CAD build for the part. Positions are in the model's coordinates, mm. A direction names the side the tool comes from. Round coordinates to 2 decimals unless told otherwise and drop trailing zeros. Loops run counter-clockwise (first coordinate to the right, second up) from the corner with the lowest first, then second, coordinate; pieces in that order, holes last. Notation, with made-up numbers: M 49,-23.5 L 96,-23.5 A31 ccw 96,15.5 Z; hole C -11,10.5 d7. An arc over 180 degrees is marked long. Use one line per item in the form item = value.
Autodesk Inventor part; units mm, degrees
ref_plane "YZ Plane" through (0, 0, 0) normal (1, 0, 0) x (0, 1, 0)
ref_plane "XZ Plane" through (0, 0, 0) normal (0, 1, 0) x (-1, 0, 0)
ref_plane "XY Plane" through (0, 0, 0) normal (0, 0, 1) x (1, 0, 0)
sketch "草圖1" plane through (0, 0, 0) normal (0, 0, 1) x (1, 0, 0)
  line L0 (-10, 120) -> (10, 120)
  line L1 (10, 120) -> (10, -20)
  line L2 (10, -20) -> (-10, -20)
  line L3 (-10, -20) -> (-10, 120)
  line L4 (10, 110) -> (-10, 110)
  line L5 (10, 120) -> (10, 110)
  line L6 (-10, 110) -> (-22, 110)
  line L7 (-22, 110) -> (-22, 120)
  line L8 (-22, 120) -> (-10, 120)
  line L9 (-10, 120) -> (-10, 110)
  line L10 (10, 110) -> (22, 110)
  line L11 (22, 110) -> (22, 120)
  line L12 (22, 120) -> (10, 120)
  line L13 (10, 120) -> (10, 110)
  point P0 (0, 0)
  point P1 (0, -20)
  dimension "d0" = 20
  dimension "d1" = 140
  dimension "d2" = 20
  dimension "d18" = 10
  dimension "d20" = 12
  dimension "d21" = 10
  dimension "d22" = 12
  dimension "d23" = 10
extrude "擠出1" add sketch "草圖1" along normal blind 10 contours L0 L1 L4 L3 | L3 L6 L7 L8 | L4 L1 L2 L3
sketch "草圖2" plane through (0, 0, 10) normal (0, 0, 1) x (1, 0, 0)
  circle A0 centre (0, 0) radius 10
  circle A1 centre (0, 0) radius 5
  dimension "d5" = 20
  dimension "d6" = 10
extrude "擠出2" add sketch "草圖2" along normal blind 10
sketch "草圖3" plane through (-10, 120, 0) normal (0, 1, 0) x (1, 0, 0)
  circle A0 centre (-2, -25) radius 10
  line L0 (20, -10) -> (-12, -10)
  line L1 (-12, 0) -> (20, 0)
  line L2 (-12, 0) -> (8, 0)
  line L3 (8, 0) -> (8, -25)
  line L4 (8, -25) -> (-12, -25)
  line L5 (-12, -25) -> (-12, 0)
  line L6 (-12, 0) -> (-12, -10)
  point P0 (10, 0)
  point P1 (0, -10)
  point P2 (0, 0)
  point P3 (32, -10)
  point P4 (32, 0)
  point P5 (8, -10)
  dimension "d9" = 20
  dimension "d10" = 25
extrude "擠出3" add sketch "草圖3" against normal blind 10 contours L4 A0 | A0 L5 L0 L3 | A0 L4
sketch "草圖4" plane through (-10, 120, 0) normal (0, 1, 0) x (1, 0, 0)
  circle A0 centre (-2, -25) radius 10
  circle A1 centre (-2, -25) radius 5
  point P0 (10, 0)
  point P1 (8, -25)
  point P2 (-12, -25)
  point P3 (0, 25)
  dimension "d13" = 10
extrude "擠出4" cut sketch "草圖4" against normal blind 10 contours A1
sketch "草圖5" plane through (0, 0, 10) normal (0, 0, 1) x (1, 0, 0)
  arc A0 (-10, 0) -> (10, 0) centre (0, 0) ccw
  line L0 (-10, 0) -> (-10, -20)
  line L1 (-10, -20) -> (10, -20)
  line L2 (10, -20) -> (10, 0)
extrude "擠出5" cut sketch "草圖5" against normal through all
equation "\"d21\" = d18"
equation "\"d22\" = d20"
equation "\"d23\" = d21"
properties part number "本體"
1. Pull direction Z, two halves, no side cores. Call faces 1 (the face through (-22, 115, 12)), 2 (the face through (2, 5, 20)), 3 (the face through (-9.693, 115.07, 29.436)): +Z half, -Z half, draft (parallel to the pull), parting line (faces both ways), or undercut.
Completed:
face_1 = draft
face_2 = +Z half
face_3 = undercut
2. Cut at D-D on y = 22. Write the cut outline in (x, z), and give its area (3 significant figures).
Completed:
outline = M -10,0 L 10,0 L 10,10 L -10,10 Z
area = 200 mm2
3. Tool access for faces 4 (the face through (-2, 115, 17)), 5 (the face through (-14, 110, 17)), 6 (the face through (0, 0, 10)): list every direction of +Z, -Z, +X, -X, +Y, -Y with a clear straight run to the whole face (end or side of a thin tool).
Completed:
face_4 = +Z, +X, +Y
face_5 = +Z, -X
face_6 = +Z
4. Cut at C-C on x = -12. Write the cut outline in (y, z), and give its area (3 significant figures).
Completed:
outline = M 110,0 L 120,0 L 120,20 L 110,20 Z; M 110,30 L 120,30 L 120,35 L 110,35 Z
area = 250 mm2
5. Probe line 1 along Z through (x, y) = (-12, 116.5); line 2 along X through (y, z) = (68.5, 5); line 3 along X through (y, z) = (115, 25). List the from-to ranges inside material, lowest first. Write a range as from..to.
Completed:
line_1 = 0..20, 30..35
line_2 = -10..10
line_3 = -22..-17, -7..-2
6. Drop flat-ended pins along their axis: P1, Ø6, axis at x = -3.5, y = 0, coming from the +Z side; P2, Ø8, axis at y = 40.5, z = 7.5, coming from the -X side; P3, Ø6, axis at x = -15.5, z = 14.5, coming from the -Y side; P4, Ø5, axis at x = -13, y = 59.5, coming from the +Z side. Give the stop position or say it passes through.
Completed:
P1 = 20
P2 = -10
P3 = 110
P4 = through
7. Cut at A-A on z = 15.5. Write the cut outline in (x, y), and give its area (3 significant figures).
Completed:
outline = M -22,110 L -2,110 L -2,120 L -22,120 Z; C 0,0 d20; hole C 0,0 d10
area = 436 mm2
8. Cut at B-B on x = 0. Write the cut outline in (y, z).
Completed:
outline = M -10,0 L 120,0 L 120,10 L 10,10 L 10,20 L 5,20 L 5,10 L -5,10 L -5,20 L -10,20 Z
